Source: CAD feature listing. Evaluate the final solid. Frame: model axes, mm. Face numbers are marked on the shaded views. A direction names the side the tool comes from. Coordinates: 2 decimals unless noted, no trailing zeros. Write each loop counter-clockwise with the first axis right and the second up, starting at its lowest first coordinate (ties: lowest second). Pieces come first, ordered by that corner, then holes. Notation, with made-up numbers: M 9,-10 L 20,-10 A18 ccw 20,4 Z; hole C 60,30 d9. An arc over 180 degrees is marked long. Answer as CSV lines item,"result". Start each with the question number.
1. Reachability of the marked faces 4, 5, 6, 7 and 8 from +Z, -Z, +X, -X, +Y, -Y: full face, straight path, thin tool, end or side. Return the list, or none.
2. Contact query for flat-ended pins moving along their axis: pin 1 Ø10 at (x, z) = (-4.5, 28) entering from -Y; pin 2 Ø5 at (x, y) = (18.5, -50) entering from +Z; pin 3 Ø6 at (x, y) = (-33.5, 81.5) entering from +Z. Output: stop coordinate, or through.
3. Section C-C on z = 14. Return the cut outline in (x, y).
4. Section B-B on y = -6.5. Return the cut outline in (x, z).
5. Line query: probe 1 along X at (y, z) = (32.5, 12); probe 2 along Y at (x, z) = (16, 38); probe 3 along Z at (x, y) = (26, -8). Output: solid intervals per line, ascending. Write a range as [from, to].
6. Mould query, pull axis Y, two halves, no side actions, for the marked faces 1, 2 and 3. Classes: pulls with the +Y half, pulls with the -Y half, needs draft (parallel to the pull), parting line crosses it, or undercut.
Autodesk Fusion 360 part; units mm, degrees
sketch "Sketch1" plane through (0, 0, 0) normal (0, 0, 1) x (1, 0, 0) in component "box"
  line L0 (40, 100) -> (-40, 100)
  line L1 (-40, 100) -> (-40, -100)
  line L2 (-40, -100) -> (40, -100)
  line L3 (40, -100) -> (40, 100)
  line L4 (40, 100) -> (-40, -100) construction
  line L5 (-40, 100) -> (40, -100) construction
  dimension "d1" = 80
  dimension "d2" = 200
extrude "Extrude1" add sketch "Sketch1" along normal blind 50 in component "box"
sketch "Sketch2" plane through (0, -100, 0) normal (0, -1, 0) x (1, 0, 0) in component "box"
  line L0 (-40, 0) -> (40, 0)
  line L1 (40, 0) -> (40, 50)
  line L2 (40, 50) -> (-40, 50)
  line L3 (-40, 50) -> (-40, 0)
  line L4 (20, 0) -> (-20, 0)
  line L5 (-20, 0) -> (-20, 20)
  line L6 (-20, 20) -> (20, 20)
  line L7 (20, 20) -> (20, 0)
  line L8 (20, 0) -> (-20, 20) construction
  line L9 (-20, 0) -> (20, 20) construction
  point P0 (0, 10)
extrude "Extrude2" cut sketch "Sketch2" against normal blind 200 contours L0 L4 L5 L6 L7 in component "box"
sketch "Sketch3" plane through (0, -100, 0) normal (0, -1, 0) x (1, 0, 0) in component "box"
  line L0 (20, 20) -> (20, 0)
  line L1 (20, 0) -> (40, 0)
  line L2 (40, 0) -> (40, 50)
  line L3 (40, 50) -> (-40, 50)
  line L4 (-40, 50) -> (-40, 0)
  line L5 (-40, 0) -> (-20, 0)
  line L6 (-20, 0) -> (-20, 20)
  line L7 (-20, 20) -> (20, 20)
  line L8 (10, 20) -> (-10, 20)
  line L9 (-10, 20) -> (-10, 40)
  line L10 (-10, 40) -> (10, 40)
  line L11 (10, 40) -> (10, 20)
  line L12 (10, 20) -> (-10, 40) construction
  line L13 (-10, 20) -> (10, 40) construction
  point P0 (0, 30)
sketch "Sketch4" plane through (40, 0, 0) normal (1, 0, 0) x (0, 1, 0) in component "box"
  line L0 (-100, 0) -> (100, 0)
  line L1 (100, 0) -> (100, 50)
  line L2 (100, 50) -> (-100, 50)
  line L3 (-100, 50) -> (-100, 0)
  line L4 (75, 30) -> (-75, 30)
  line L5 (-75, 30) -> (-75, 50)
  line L6 (-75, 50) -> (75, 50)
  line L7 (75, 50) -> (75, 30)
  line L8 (75, 30) -> (-75, 50) construction
  line L9 (-75, 30) -> (75, 50) construction
  point P0 (0, 40)
extrude "Extrude3" cut sketch "Sketch4" against normal blind 80 contours L2 L4 L5 L6 L7 in component "box"
extrude "Extrude4" add sketch "Sketch3" against normal blind 200 contours L7 L8 L9 L10 L11 in component "box"
sketch "Sketch5" plane through (0, -100, 0) normal (0, -1, 0) x (1, 0, 0) in component "box"
  line L0 (-20, 20) -> (20, 20)
  line L1 (20, 20) -> (20, 0)
  line L2 (20, 0) -> (40, 0)
  line L3 (40, 0) -> (40, 50)
  line L4 (40, 50) -> (-40, 50)
  line L5 (-40, 50) -> (-40, 0)
  line L6 (-40, 0) -> (-20, 0)
  line L7 (-20, 0) -> (-20, 20)
  line L8 (10, 20) -> (-10, 20)
  line L9 (-10, 20) -> (-10, 40)
  line L10 (-10, 40) -> (10, 40)
  line L11 (10, 40) -> (10, 20)
  line L12 (10, 20) -> (-10, 40) construction
  line L13 (-10, 20) -> (10, 40) construction
  point P0 (0, 30)
extrude "Extrude5" cut sketch "Sketch5" against normal blind 25 contours L0 L8 L9 L10 L11 in component "box"
sketch "Sketch6" plane through (0, 100, 0) normal (0, 1, 0) x (-1, 0, 0) in component "box"
  line L0 (-20, 20) -> (20, 20)
  line L1 (20, 20) -> (20, 0)
  line L2 (20, 0) -> (40, 0)
  line L3 (40, 0) -> (40, 50)
  line L4 (40, 50) -> (-40, 50)
  line L5 (-40, 50) -> (-40, 0)
  line L6 (-40, 0) -> (-20, 0)
  line L7 (-20, 0) -> (-20, 20)
  line L8 (10, 20) -> (-10, 20)
  line L9 (-10, 20) -> (-10, 40)
  line L10 (-10, 40) -> (10, 40)
  line L11 (10, 40) -> (10, 20)
  line L12 (10, 20) -> (-10, 40) construction
  line L13 (-10, 20) -> (10, 40) construction
  point P0 (0, 30)
extrude "Extrude6" cut sketch "Sketch6" against normal blind 25 contours L0 L8 L9 L10 L11 in component "box"
sketch "Sketch7" plane through (40, 0, 0) normal (1, 0, 0) x (0, 1, 0) in component "box"
  line L0 (75, 50) -> (75, 30)
  line L1 (75, 30) -> (-75, 30)
  line L2 (-75, 30) -> (-75, 50)
  line L3 (-75, 50) -> (-100, 50)
  line L4 (-100, 50) -> (-100, 0)
  line L5 (-100, 0) -> (100, 0)
  line L6 (100, 0) -> (100, 50)
  line L7 (100, 50) -> (75, 50)
  circle A0 centre (-75, 50) radius 20
extrude "Extrude7" add sketch "Sketch7" against normal blind 80 contours L2 L3 A0 picked at (-86.5147, 56.648) in component "box"
sketch "Sketch8" plane through (0, 100, 0) normal (0, 1, 0) x (-1, 0, 0) in component "box"
  line L0 (10, 40) -> (10, 20)
  line L1 (10, 20) -> (20, 20)
  line L2 (20, 20) -> (20, 0)
  line L3 (20, 0) -> (40, 0)
  line L4 (40, 0) -> (40, 50)
  line L5 (40, 50) -> (-40, 50)
  line L6 (-40, 50) -> (-40, 0)
  line L7 (-40, 0) -> (-20, 0)
  line L8 (-20, 0) -> (-20, 20)
  line L9 (-20, 20) -> (-10, 20)
  line L10 (-10, 20) -> (-10, 40)
  line L11 (-10, 40) -> (10, 40)
  circle A0 centre (0.1969, 50) radius 19.8031
extrude "Extrude8" add sketch "Sketch8" against normal blind 25 contours L5 A0 in component "box"
sketch "Sketch9" plane through (40, 0, 0) normal (1, 0, 0) x (0, 1, 0) in component "box"
  line L0 (75, 50) -> (75, 30)
  line L1 (75, 30) -> (-75, 30)
  arc A0 (-75, 30) -> (-95, 50) centre (-75, 50) ccw
  line L2 (-95, 50) -> (-100, 50)
  line L3 (-100, 50) -> (-100, 0)
  line L4 (-100, 0) -> (100, 0)
  line L5 (100, 0) -> (100, 50)
  line L6 (100, 50) -> (75, 50)
  line L7 (75, 30) -> (-75, 30)
  line L8 (-75, 30) -> (-75, 70)
  line L9 (-75, 70) -> (75, 70)
  line L10 (75, 70) -> (75, 30)
  line L11 (75, 30) -> (-75, 70) construction
  line L12 (-75, 30) -> (75, 70) construction
  point P0 (0, 50)
extrude "Extrude9" cut sketch "Sketch9" against normal blind 80 contours A0 L8 in component "box"
sketch "Sketch10" plane through (0, -100, 0) normal (0, -1, 0) x (1, 0, 0) in component "box"
  line L0 (10, 40) -> (10, 20)
  line L1 (10, 20) -> (20, 20)
  line L2 (20, 20) -> (20, 0)
  line L3 (20, 0) -> (40, 0)
  line L4 (40, 0) -> (40, 50)
  line L5 (40, 50) -> (-40, 50)
  line L6 (-40, 50) -> (-40, 0)
  line L7 (-40, 0) -> (-20, 0)
  line L8 (-20, 0) -> (-20, 20)
  line L9 (-20, 20) -> (-10, 20)
  line L10 (-10, 20) -> (-10, 40)
  line L11 (-10, 40) -> (10, 40)
  line L12 (10, 20) -> (-10, 20)
  line L13 (-10, 20) -> (-10, 40)
  line L14 (-10, 40) -> (10, 40)
  line L15 (10, 40) -> (10, 20)
  line L16 (10, 20) -> (-10, 40) construction
  line L17 (-10, 20) -> (10, 40) construction
  point P0 (0, 30)
extrude "Extrude10" add sketch "Sketch10" against normal blind 50 contours L0 L10 L11 L12 L13 L14 L15 in component "box"
sketch "Sketch11" plane through (0, -100, 0) normal (0, -1, 0) x (1, 0, 0) in component "box"
  line L0 (-20, 20) -> (20, 20)
  line L1 (20, 20) -> (20, 0)
  line L2 (20, 0) -> (40, 0)
  line L3 (40, 0) -> (40, 50)
  line L4 (40, 50) -> (-40, 50)
  line L5 (-40, 50) -> (-40, 0)
  line L6 (-40, 0) -> (-20, 0)
  line L7 (-20, 0) -> (-20, 20)
  line L8 (10, 20) -> (-10, 20)
  line L9 (-10, 20) -> (-10, 40)
  line L10 (-10, 40) -> (10, 40)
  line L11 (10, 40) -> (10, 20)
  line L12 (10, 20) -> (-10, 40) construction
  line L13 (-10, 20) -> (10, 40) construction
  point P0 (0, 30)
extrude "Extrude11" cut sketch "Sketch11" against normal blind 25 contours L0 L8 L9 L10 L11 in component "box"
component "box" placed x (1, 0, 0) y (0, 1, 0) z (0, 0, 1) at (0, 0, 0)
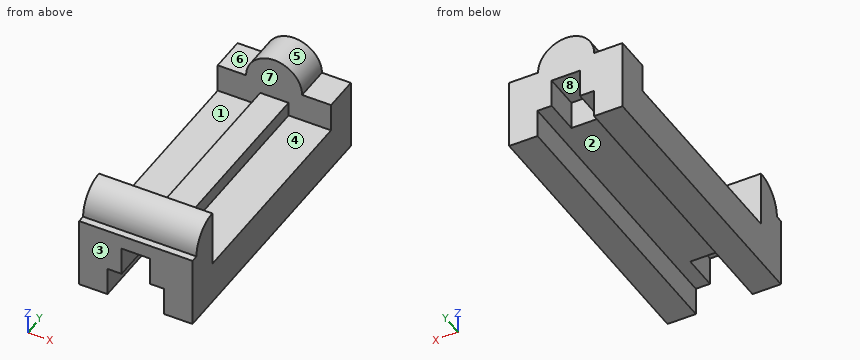
Values:
1,face 4,"+Z, +X"
1,face 5,"+Z, +Y"
1,face 6,"+Z, -X, +Y"
1,face 7,"+Z"
1,face 8,"-Z, +Y"
2,pin 1,"y = -75"
2,pin 2,"z = 30"
2,pin 3,"z = 50"
3,outline,"M -40,-100 L -20,-100 L -20,100 L -40,100 Z; M 20,-100 L 40,-100 L 40,100 L 20,100 Z"
4,outline,"M -40,0 L -20,0 L -20,20 L 20,20 L 20,0 L 40,0 L 40,30 L 10,30 L 10,40 L -10,40 L -10,30 L -40,30 Z"
5,probe 1,"[-40, -20], [20, 40]"
5,probe 2,"[-100, -75], [75, 100]"
5,probe 3,"[0, 30]"
6,face 1,"undercut"
6,face 2,"needs draft"
6,face 3,"pulls with the -Y half"
